from build123d import *

# Parameters (mm, degrees)
SKETCH009_W     = 96
SKETCH009_H     = 76
PAD004_DEPTH    = 4
SKETCH012_R     = 28.5
POCKET002_DEPTH = 0.8
SKETCH010_R     = 1.5
HOLE003_DEPTH   = 4.001


with BuildPart() as part:
    # Sketch009 → Pad004 (new body)
    with BuildSketch(Plane.YZ.offset(126)):
        with Locations((-48, 38)):
            Rectangle(SKETCH009_W, SKETCH009_H)
    extrude(amount=PAD004_DEPTH)

    # Sketch012 (on Face4 of Hole003) → Pocket002 (cut)
    with BuildSketch(Plane(origin=(126, 0, 0), x_dir=(0, 1, 0), z_dir=(-1, 0, 0))):
        with Locations((-50, -38)):
            Circle(SKETCH012_R)
    extrude(amount=-POCKET002_DEPTH, mode=Mode.SUBTRACT)

    # Sketch010 (on Face6 of Pad004) → Hole003 (cut, through all)
    with BuildSketch(Plane.YZ.offset(130)):
        with Locations((-50, 65)):
            Circle(SKETCH010_R)
        with Locations((-43.9919347832, 64.3230536289)):
            Circle(SKETCH010_R)
        with Locations((-38.2851390438, 62.3261594334)):
            Circle(SKETCH010_R)
        with Locations((-33.1657753498, 59.1094500266)):
            Circle(SKETCH010_R)
        with Locations((-28.8905499734, 54.8342246502)):
            Circle(SKETCH010_R)
        with Locations((-25.6738405666, 49.7148609562)):
            Circle(SKETCH010_R)
        with Locations((-23.6769463711, 44.0080652168)):
            Circle(SKETCH010_R)
        with Locations((-23, 38)):
            Circle(SKETCH010_R)
        with Locations((-23.6769463711, 31.9919347832)):
            Circle(SKETCH010_R)
        with Locations((-25.6738405666, 26.2851390438)):
            Circle(SKETCH010_R)
        with Locations((-28.8905499734, 21.1657753498)):
            Circle(SKETCH010_R)
        with Locations((-33.1657753498, 16.8905499734)):
            Circle(SKETCH010_R)
        with Locations((-38.2851390438, 13.6738405666)):
            Circle(SKETCH010_R)
        with Locations((-43.9919347832, 11.6769463711)):
            Circle(SKETCH010_R)
        with Locations((-50, 11)):
            Circle(SKETCH010_R)
        with Locations((-56.0080652168, 11.6769463711)):
            Circle(SKETCH010_R)
        with Locations((-61.7148609562, 13.6738405666)):
            Circle(SKETCH010_R)
        with Locations((-66.8342246502, 16.8905499734)):
            Circle(SKETCH010_R)
        with Locations((-71.1094500266, 21.1657753498)):
            Circle(SKETCH010_R)
        with Locations((-74.3261594334, 26.2851390438)):
            Circle(SKETCH010_R)
        with Locations((-76.3230536289, 31.9919347832)):
            Circle(SKETCH010_R)
        with Locations((-77, 38)):
            Circle(SKETCH010_R)
        with Locations((-76.3230536289, 44.0080652168)):
            Circle(SKETCH010_R)
        with Locations((-74.3261594334, 49.7148609562)):
            Circle(SKETCH010_R)
        with Locations((-71.1094500266, 54.8342246502)):
            Circle(SKETCH010_R)
        with Locations((-66.8342246502, 59.1094500266)):
            Circle(SKETCH010_R)
        with Locations((-61.7148609562, 62.3261594334)):
            Circle(SKETCH010_R)
        with Locations((-56.0080652168, 64.3230536289)):
            Circle(SKETCH010_R)
        with Locations((-47.4248170496, 60.8553808275)):
            Circle(SKETCH010_R)
        with Locations((-42.403581575, 59.7093165971)):
            Circle(SKETCH010_R)
        with Locations((-37.7632622401, 57.4746565823)):
            Circle(SKETCH010_R)
        with Locations((-33.7365440327, 54.2634559673)):
            Circle(SKETCH010_R)
        with Locations((-30.5253434177, 50.2367377599)):
            Circle(SKETCH010_R)
        with Locations((-28.2906834029, 45.596418425)):
            Circle(SKETCH010_R)
        with Locations((-27.1446191725, 40.5751829504)):
            Circle(SKETCH010_R)
        with Locations((-27.1446191725, 35.4248170496)):
            Circle(SKETCH010_R)
        with Locations((-28.2906834029, 30.403581575)):
            Circle(SKETCH010_R)
        with Locations((-30.5253434177, 25.7632622401)):
            Circle(SKETCH010_R)
        with Locations((-33.7365440327, 21.7365440327)):
            Circle(SKETCH010_R)
        with Locations((-37.7632622401, 18.5253434177)):
            Circle(SKETCH010_R)
        with Locations((-42.403581575, 16.2906834029)):
            Circle(SKETCH010_R)
        with Locations((-47.4248170496, 15.1446191725)):
            Circle(SKETCH010_R)
        with Locations((-52.5751829504, 15.1446191725)):
            Circle(SKETCH010_R)
        with Locations((-57.596418425, 16.2906834029)):
            Circle(SKETCH010_R)
        with Locations((-62.2367377599, 18.5253434177)):
            Circle(SKETCH010_R)
        with Locations((-66.2634559673, 21.7365440327)):
            Circle(SKETCH010_R)
        with Locations((-69.4746565823, 25.7632622401)):
            Circle(SKETCH010_R)
        with Locations((-71.7093165971, 30.403581575)):
            Circle(SKETCH010_R)
        with Locations((-72.8553808275, 35.4248170496)):
            Circle(SKETCH010_R)
        with Locations((-72.8553808275, 40.5751829504)):
            Circle(SKETCH010_R)
        with Locations((-71.7093165971, 45.596418425)):
            Circle(SKETCH010_R)
        with Locations((-69.4746565823, 50.2367377599)):
            Circle(SKETCH010_R)
        with Locations((-66.2634559673, 54.2634559673)):
            Circle(SKETCH010_R)
        with Locations((-62.2367377599, 57.4746565823)):
            Circle(SKETCH010_R)
        with Locations((-57.596418425, 59.7093165971)):
            Circle(SKETCH010_R)
        with Locations((-52.5751829504, 60.8553808275)):
            Circle(SKETCH010_R)
        with Locations((-50, 57)):
            Circle(SKETCH010_R)
        with Locations((-41.7562089568, 55.1184084901)):
            Circle(SKETCH010_R)
        with Locations((-35.1452018331, 49.8463062353)):
            Circle(SKETCH010_R)
        with Locations((-31.4763696685, 42.2278977452)):
            Circle(SKETCH010_R)
        with Locations((-31.4763696685, 33.7721022548)):
            Circle(SKETCH010_R)
        with Locations((-35.1452018331, 26.1536937647)):
            Circle(SKETCH010_R)
        with Locations((-41.7562089568, 20.8815915099)):
            Circle(SKETCH010_R)
        with Locations((-50, 19)):
            Circle(SKETCH010_R)
        with Locations((-58.2437910432, 20.8815915099)):
            Circle(SKETCH010_R)
        with Locations((-64.8547981669, 26.1536937647)):
            Circle(SKETCH010_R)
        with Locations((-68.5236303315, 33.7721022548)):
            Circle(SKETCH010_R)
        with Locations((-68.5236303315, 42.2278977452)):
            Circle(SKETCH010_R)
        with Locations((-64.8547981669, 49.8463062353)):
            Circle(SKETCH010_R)
        with Locations((-58.2437910432, 55.1184084901)):
            Circle(SKETCH010_R)
        with Locations((-46.5509255237, 53.1113826388)):
            Circle(SKETCH010_R)
        with Locations((-40.3359080712, 50.1183879783)):
            Circle(SKETCH010_R)
        with Locations((-36.0349825475, 44.7251979563)):
            Circle(SKETCH010_R)
        with Locations((-34.5, 38)):
            Circle(SKETCH010_R)
        with Locations((-36.0349825475, 31.2748020437)):
            Circle(SKETCH010_R)
        with Locations((-40.3359080712, 25.8816120217)):
            Circle(SKETCH010_R)
        with Locations((-46.5509255237, 22.8886173612)):
            Circle(SKETCH010_R)
        with Locations((-53.4490744763, 22.8886173612)):
            Circle(SKETCH010_R)
        with Locations((-59.6640919288, 25.8816120217)):
            Circle(SKETCH010_R)
        with Locations((-63.9650174525, 31.2748020437)):
            Circle(SKETCH010_R)
        with Locations((-65.5, 38)):
            Circle(SKETCH010_R)
        with Locations((-63.9650174525, 44.7251979563)):
            Circle(SKETCH010_R)
        with Locations((-59.6640919288, 50.1183879783)):
            Circle(SKETCH010_R)
        with Locations((-53.4490744763, 53.1113826388)):
            Circle(SKETCH010_R)
        with Locations((-50, 50)):
            Circle(SKETCH010_R)
        with Locations((-40.6180222104, 45.4818776223)):
            Circle(SKETCH010_R)
        with Locations((-38.3008650538, 35.3297487925)):
            Circle(SKETCH010_R)
        with Locations((-44.7933951306, 27.1883735852)):
            Circle(SKETCH010_R)
        with Locations((-55.2066048694, 27.1883735852)):
            Circle(SKETCH010_R)
        with Locations((-61.6991349462, 35.3297487925)):
            Circle(SKETCH010_R)
        with Locations((-59.3819777896, 45.4818776223)):
            Circle(SKETCH010_R)
        with Locations((-46.7458719566, 44.7572665093)):
            Circle(SKETCH010_R)
        with Locations((-42.6880406586, 39.6689070047)):
            Circle(SKETCH010_R)
        with Locations((-44.1362638815, 33.3238264861)):
            Circle(SKETCH010_R)
        with Locations((-50, 30.5)):
            Circle(SKETCH010_R)
        with Locations((-55.8637361185, 33.3238264861)):
            Circle(SKETCH010_R)
        with Locations((-57.3119593414, 39.6689070047)):
            Circle(SKETCH010_R)
        with Locations((-53.2541280434, 44.7572665093)):
            Circle(SKETCH010_R)
        with Locations((-50, 38)):
            Circle(SKETCH010_R)
    extrude(amount=-HOLE003_DEPTH, mode=Mode.SUBTRACT)


solid = part.part
The model under review builds one solid part; all positions refer to its coordinate system, in mm. A direction names the side the tool comes from. Coordinates: 2 decimals unless noted, no trailing zeros. Use a Markdown table: item, result. Add a question column.
1. Clearance check with flat-ended pins moving along their axes: pin 1 Ø3.5 at (y, z) = (-30.53, 50.24) entering from -X; pin 2 Ø1.8 at (y, z) = (-37.76, 57.47) entering from -X. State where each tip first meets the part, or that it passes through.
2. Draft analysis for pull direction Z (two halves, no side actions). For faces 1 (the face through (128, -96, 37)), 2 (the face through (128.422, -45.994, 15.595)), state which applies: pulls with the +Z half, pulls with the -Z half, needs draft (parallel to the pull), parting line crosses it, or undercut.
3. Add section A-A on x = 129. Give the number of separate pieces and of enclosed holes in the cut face, plus the area to 3 significant figures.
4. To check wall thickness, follow line 1 (Y direction, x = 128.6, z = 41.5); line 2 (Y direction, x = 128, z = 23.5); line 3 (Y direction, x = 127, z = 52). State the ranges of each line that lie inside material, in increasing order.
5. Machinability: for faces 3 (the face through (126.8, -44, 38)), 4 (the face through (128.42, -57.2, 63.41)), which of the approach directions +Z, -Z, +X, -X, +Y, -Y give a long, thin tool a straight path to every point of the face, cutting with its end or side? Answer none if there is none.
Returned:
| question | item | result |
|---|---|---|
| 1 | pin 1 | stops at x = 126.8 |
| 1 | pin 2 | passes through |
| 2 | face 1 | needs draft |
| 2 | face 2 | undercut |
| 3 | separate pieces | 1 |
| 3 | enclosed holes | 99 |
| 3 | area | 6,600 mm² |
| 4 | line 1 | y = -96 to -74.04, -71.67 to -69.84, -67.21 to -32.79, -30.16 to -28.33, -25.96 to 0 |
| 4 | line 2 | y = -96 to -54.82, -52.08 to -47.92, -45.18 to 0 |
| 4 | line 3 | y = -96 to -54.46, -52.44 to -47.56, -45.54 to 0 |
| 5 | face 3 | -X |
| 5 | face 4 | +X, -X |
